Geometry: see drawing. Coordinates: mm, zero at the bounding-box minimum. A direction names the side the tool comes from. Round coordinates to 2 decimals unless told otherwise and drop trailing zeros. Write each loop counter-clockwise with the first axis right and the second up, starting at its lowest first coordinate (ties: lowest second). Pieces come first, ordered by that corner, then holes. Notation, with made-up numbers: (31, 65.25) - (55, 65.25) arc R14 ccw to (55, 85.25) - close; hole circle Ø1 at (62.25, -21.5). An arc over 180 degrees is marked (long way). Use a Markdown table: item, result. Add a question column.
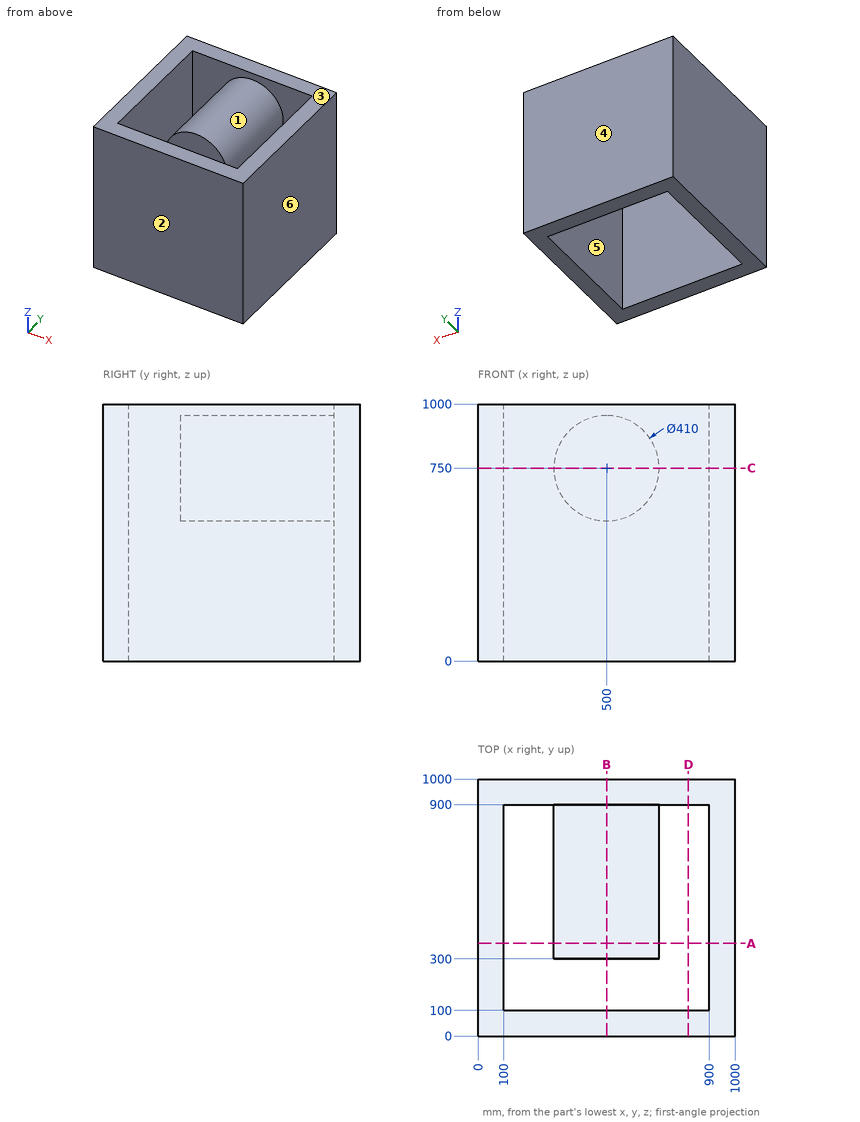
1) Section B-B, the plane x = 500. Return the cut outline in (y, z).
2) Section D-D, the plane x = 819. Return the cut outline in (y, z), then the cut area to 3 significant figures.
3) Material intervals for L1, parallel to X at y = 772, z = 130; L2, parallel to X at y = 716.5, z = 690, sorted ascending. Write a range as from..to.
4) Section A-A, the plane y = 360. Return the cut outline in (x, z), then the cut area to 3 significant figures.
5) Section C-C, the plane z = 750. Return the cut outline in (x, y), then the cut area to 3 significant figures.
6) Draft query along Y for the marked faces 1, 2, 3 and 4. Return one class per face: released by +Y, released by -Y, zero draft, split by the parting line, or undercut.
7) Set-up query: the marked faces 5 and 6. Return all of +Z, -Z, +X, -X, +Y, -Y with unobstructed straight access to the full face (end or side cutting, diameter ignored); none if empty.
Output values:
| question | item | result |
|---|---|---|
| 1 | outline | (0, 0) - (100, 0) - (100, 1000) - (0, 1000) - close; (300, 545) - (900, 545) - (900, 0) - (1000, 0) - (1000, 1000) - (900, 1000) - (900, 955) - (300, 955) - close |
| 2 | outline | (0, 0) - (100, 0) - (100, 1000) - (0, 1000) - close; (900, 0) - (1000, 0) - (1000, 1000) - (900, 1000) - close |
| 2 | area | 200,000 mm^2 |
| 3 | L1 | x = 0..100, 900..1000 |
| 3 | L2 | x = 0..100, 303.98..696.02, 900..1000 |
| 4 | outline | (0, 0) - (100, 0) - (100, 1000) - (0, 1000) - close; circle Ø410 at (500, 750); (900, 0) - (1000, 0) - (1000, 1000) - (900, 1000) - close |
| 4 | area | 332,000 mm^2 |
| 5 | outline | (0, 0) - (1000, 0) - (1000, 1000) - (0, 1000) - close; hole (100, 100) - (900, 100) - (900, 900) - (705, 900) - (705, 300) - (295, 300) - (295, 900) - (100, 900) - close |
| 5 | area | 606,000 mm^2 |
| 6 | face 1 | undercut |
| 6 | face 2 | released by -Y |
| 6 | face 3 | zero draft |
| 6 | face 4 | released by +Y |
| 7 | face 5 | +Z, -Z |
| 7 | face 6 | +Z, -Z, +X, +Y, -Y |
